Part print with two shaded views. Sizes in mm from the minimum x, y, z corner. Coordinates: 2 decimals unless noted, no trailing zeros. Loops run counter-clockwise (first coordinate to the right, second up) from the corner with the lowest first, then second, coordinate; pieces in that order, holes last. Notation, with made-up numbers: (76.5, 23.25) -> (129.5, 23.25) arc R28 ccw to (129.5, 59.25) -> close; hole circle Ø6 at (18.5, -29.5). An arc over 180 degrees is marked (long way). Write each question's results on one line, items separated by ' | '.
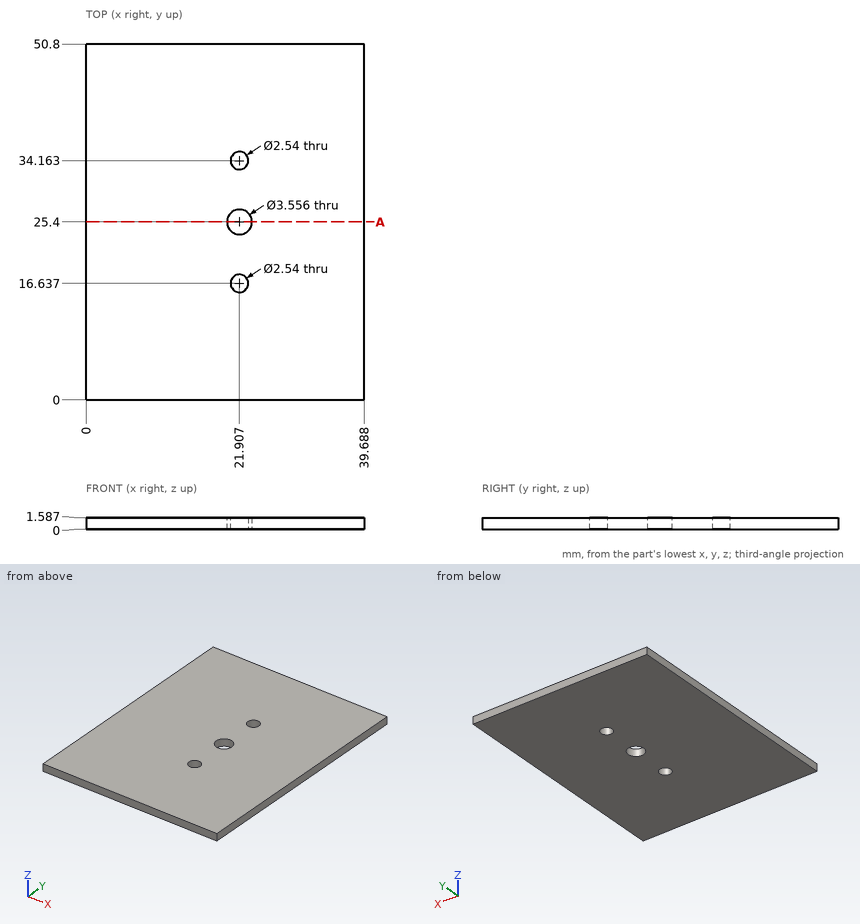
Q1. Cut at A-A on y = 25.4. Write the cut outline in (x, z) (1 decimal).
Results are:
outline: (0, 0) -> (20.1, 0) -> (20.1, 1.6) -> (0, 1.6) -> close; (23.7, 0) -> (39.7, 0) -> (39.7, 1.6) -> (23.7, 1.6) -> close
Q2. Drop a flat-ended pin along its axis: pin 1 (2 mm diameter, centred on x = 10.5, y = 6, fed in from -Z). Give the stop position or say it passes through.
Results are:
pin 1: z = 0
Q3. Wall check: L1, parallel to Y at x = 22, z = 0.85 (1 decimal); L2, parallel to X at y = 34, z = 0.65; L3, parallel to X at y = 24, z = 1.05 (1 decimal). Give the ranges that are in metal, low to high. Write a range as from..to.
Results are:
L1: 0..15.4, 17.9..23.6, 27.2..32.9, 35.4..50.8 | L2: 0..20.65, 23.17..39.69 | L3: 0..20.8, 23..39.7
